Read the model definition and answer for the solid it produces. Units are mm, in the model's axes. Round coordinates to 2 decimals unless told otherwise and drop trailing zeros. Order: outer loops, then holes, each group sorted by start corner. A loop starts at its lowest first (then second) coordinate and runs counter-clockwise, first axis right, second up. Notation, with made-up numbers: (10.5, 72.25) - (20.5, 72.25) arc R26 ccw to (20.5, 111.25) - close; hole circle Ø5 at (75.5, 19.25). An arc over 180 degrees is marked (long way). Put each result on its own line as item: value. Start each with the question number.
Q1. Section B-B on x = 1 is taken. Give the vertices of the cut face in (y, z), then the cut area to 3 significant figures.
Q2. For a pull along Z with two mould halves and no side action, classify faces 1 (the face through (5.261, -31.247, -8.552)), 2 (the face through (8.327, -34, -2)), 3 (the face through (-1.81, -38.41, -5.76)) as pulls with the +Z half, pulls with the -Z half, needs draft (parallel to the pull), parting line crosses it, or undercut.
Q3. Section A-A on y = -32.75 is taken. State how many separate pieces and enclosed holes the cut face has, then the cut area to 3 significant figures.
Q4. Section D-D on x = -1.25 is taken. Give the vertices of the cut face in (y, z).
Q5. Section C-C on x = 5.5 is taken. Give the vertices of the cut face in (y, z).
Q6. Each of these flat-tipped pins is pushed along its axis until it touches: pin 1 Ø6 at (y, z) = (-32.55, -4.46) entering from +X; pin 2 Ø1.5 at (x, y) = (4, -35) entering from -Z; pin 3 Ø4 at (x, z) = (0.5, 0) entering from +Y; pin 4 Ø2 at (x, y) = (2, -35.5) entering from -Z. Where does it stop, or does it pass through?
Q7. Find the intervals of material crossed by line 1 along Z through (x, y) = (2.25, -32); line 2 along Y through (x, z) = (7.75, -3.25); line 3 along Z through (x, y) = (-0.75, -31.5) (3 decimals), in increasing order. Write a range as from..to.
from build123d import *

# Parameters (mm, degrees)
F_5_0_5_DIAMETER_HOLE1_D      = 5
F_3_0_3_DIAMETER_HOLE1_REACH  = 17.726
F_3_0_3_DIAMETER_HOLE1_BORE_R = 1.5


with BuildPart() as part:
    # Sketch1 → Revolve1 (revolve)
    with BuildSketch(Plane(origin=(0, 0, -4.458227774), x_dir=(-1, 0, 0), z_dir=(0, 0, -1)), mode=Mode.PRIVATE) as revolve1_sk:
        with BuildLine():
            Line((-8.327233411, -26.554384432), (-8.327233411, -32.554384432))
            Line((-8.327233411, -32.554384432), (2.672766589, -32.554384432))
            Line((2.672766589, -32.554384432), (2.672766589, -26.554384432))
            Line((2.672766589, -26.554384432), (0.968480701, -26.554384432))
            ThreePointArc((0.968480701, -26.554384432), (-0.502233411, -27.054384432), (-1.972947524, -26.554384432))
            Line((-1.972947524, -26.554384432), (-8.327233411, -26.554384432))
        make_face()
    revolve(revolve1_sk.sketch.rotate(Axis((8.327233411, -32.554384432, -4.458227774), (-1, 0, 0)), 270), axis=Axis((8.327233411, -32.554384432, -4.458227774), (-1, 0, 0)))

    # Ø5.0 (5) Diameter Hole1 (through all)
    with Locations(Plane.ZY.offset(2.672766589)):
        with Locations((-4.458227774, -32.554384432)):
            Hole(F_5_0_5_DIAMETER_HOLE1_D / 2)

    # Ø3.0 (3) Diameter Hole1 bore (on position points) → Ø3.0 (3) Diameter Hole1 (cut, up to next)
    with BuildSketch(Plane(origin=(5.327233411, -32.836401262, -10.451596318), x_dir=(0, -0.998894757378, 0.047002805043), z_dir=(0, -0.047002805043, -0.998894757378)), mode=Mode.PRIVATE) as f_3_0_3_diameter_hole1_sk1:
        Circle(F_3_0_3_DIAMETER_HOLE1_BORE_R)
    f_3_0_3_diameter_hole1_tool1 = extrude(f_3_0_3_diameter_hole1_sk1.sketch, amount=-F_3_0_3_DIAMETER_HOLE1_REACH, mode=Mode.PRIVATE) & part.part
    add(f_3_0_3_diameter_hole1_tool1.solids().sort_by_distance((5.327233, -32.836401, -10.451596))[0], mode=Mode.SUBTRACT)


solid = part.part
Findings:
1. outline: circle Ø11.1 at (-32.55, -4.46); hole circle Ø5 at (-32.55, -4.46)
1. area: 77.2 mm2
2. face 1: undercut
2. face 2: needs draft
2. face 3: parting line crosses it
3. separate pieces: 3
3. enclosed holes: 0
3. area: 64.6 mm2
4. outline: circle Ø12 at (-32.55, -4.46); hole circle Ø5 at (-32.55, -4.46)
5. outline: (-34.32, -10.19) - (-34.14, -6.39) arc R2.5 cw (long way) to (-31.16, -6.53) - (-31.34, -10.33) arc R6 ccw (long way) to start
6. pin 1: x = 8.33
6. pin 2: z = -10.21
6. pin 3: y = -27.42
6. pin 4: z = -10.13
7. line 1: -10.43..-6.9, -2.02..1.52
7. line 2: -38.43..-34.74, -30.37..-26.68
7. line 3: -10.213..-6.725, -2.191..1.296
